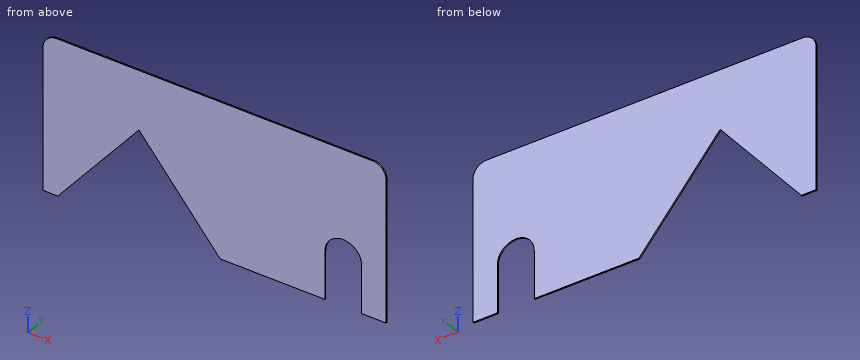
from build123d import *

# Parameters (mm, degrees)
SKETCH1_W          = 104.4
SKETCH1_H          = 0.9
BASE_FLANGE1_DEPTH = 116.2
FILLET1_R          = 9.2
CUT_EXTRUDE1_DEPTH = 128.389520762
CUT_EXTRUDE2_DEPTH = 128.389520762


# Sheet-metal steps are written as plain solids
with BuildPart() as part:
    # Sketch1 → Base-Flange1 (new, symmetric)
    with BuildSketch(Plane(origin=(0, 0, 0), x_dir=(0, 0, -1), z_dir=(1, 0, 0))):
        with Locations((0, -0.45)):
            Rectangle(SKETCH1_W, SKETCH1_H)
    extrude(amount=BASE_FLANGE1_DEPTH, both=True)

    # Fillet1
    fillet1_edges = [part.edges().sort_by_distance(p)[0] for p in [
        (116.2, -0.45, 52.2),
        (-116.2, -0.45, 52.2),
    ]]
    fillet(fillet1_edges, radius=FILLET1_R)

    # Sketch2 → Cut-Extrude1 (cut, through all)
    with BuildSketch(Plane(origin=(0, 0, 0), x_dir=(1, 0, 0), z_dir=(0, 1, 0))):
        with BuildLine():
            Line((74.7, 52.2), (99.7, 52.2))
            Line((99.7, 52.2), (99.7, 20.2))
            ThreePointArc((99.7, 20.2), (87.2, 7.7), (74.7, 20.2))
            Line((74.7, 20.2), (74.7, 52.2))
        make_face()
    extrude(amount=-CUT_EXTRUDE1_DEPTH, mode=Mode.SUBTRACT)

    # Sketch3 → Cut-Extrude2 (cut, through all)
    with BuildSketch(Plane(origin=(0, 0, 0), x_dir=(1, 0, 0), z_dir=(0, 1, 0))):
        Polygon((-106.2, 52.2), (-51.2, -12.607406984), (3.8, 52.2), align=None)
    extrude(amount=-CUT_EXTRUDE2_DEPTH, mode=Mode.SUBTRACT)


solid = part.part
Input: part model. Units: mm. Frame: model coordinates. Round coordinates to 2 decimals unless told otherwise and drop trailing zeros. Order: outer loops, then holes, each group sorted by start corner. A loop starts at its lowest first (then second) coordinate and runs counter-clockwise, first axis right, second up.
1. Cut plane B-B, the plane z = -36. Output: boundary loops of the cut face in (x, y), then the cut area to 3 significant figures.
The answers:
outline: (-116.2, -0.9) - (-92.45, -0.9) - (-92.45, 0) - (-116.2, 0) - close; (-9.95, -0.9) - (74.7, -0.9) - (74.7, 0) - (-9.95, 0) - close; (99.7, -0.9) - (116.2, -0.9) - (116.2, 0) - (99.7, 0) - close
area: 112 mm2
2. Material intervals for line 1 (X direction, y = -0.6, z = -30.5); line 2 (X direction, y = -0.35, z = -22); line 3 (X direction, y = -0.3, z = 2.5), sorted ascending.
The answers:
line 1: x = -116.2 to -87.78, -14.62 to 74.7, 99.7 to 116.2
line 2: x = -116.2 to -80.57, -21.83 to 74.7, 99.7 to 116.2
line 3: x = -116.2 to -59.78, -42.62 to 116.2
3. Cut plane C-C, the plane x = 87.2. Output: boundary loops of the cut face in (y, z).
The answers:
outline: (-0.9, -7.7) - (0, -7.7) - (0, 52.2) - (-0.9, 52.2) - close
4. Cut plane A-A, the plane y = -0.55. Output: boundary loops of the cut face in (x, z).
The answers:
outline: (-116.2, -52.2) - (-106.2, -52.2) - (-51.2, 12.61) - (3.8, -52.2) - (74.7, -52.2) - (74.7, -20.2) arc R12.5 cw to (99.7, -20.2) - (99.7, -52.2) - (116.2, -52.2) - (116.2, 43) arc R9.2 ccw to (107, 52.2) - (-107, 52.2) arc R9.2 ccw to (-116.2, 43) - close
5. Cut plane D-D, the plane x = -33. Output: boundary loops of the cut face in (y, z).
The answers:
outline: (-0.9, -8.84) - (0, -8.84) - (0, 52.2) - (-0.9, 52.2) - close
